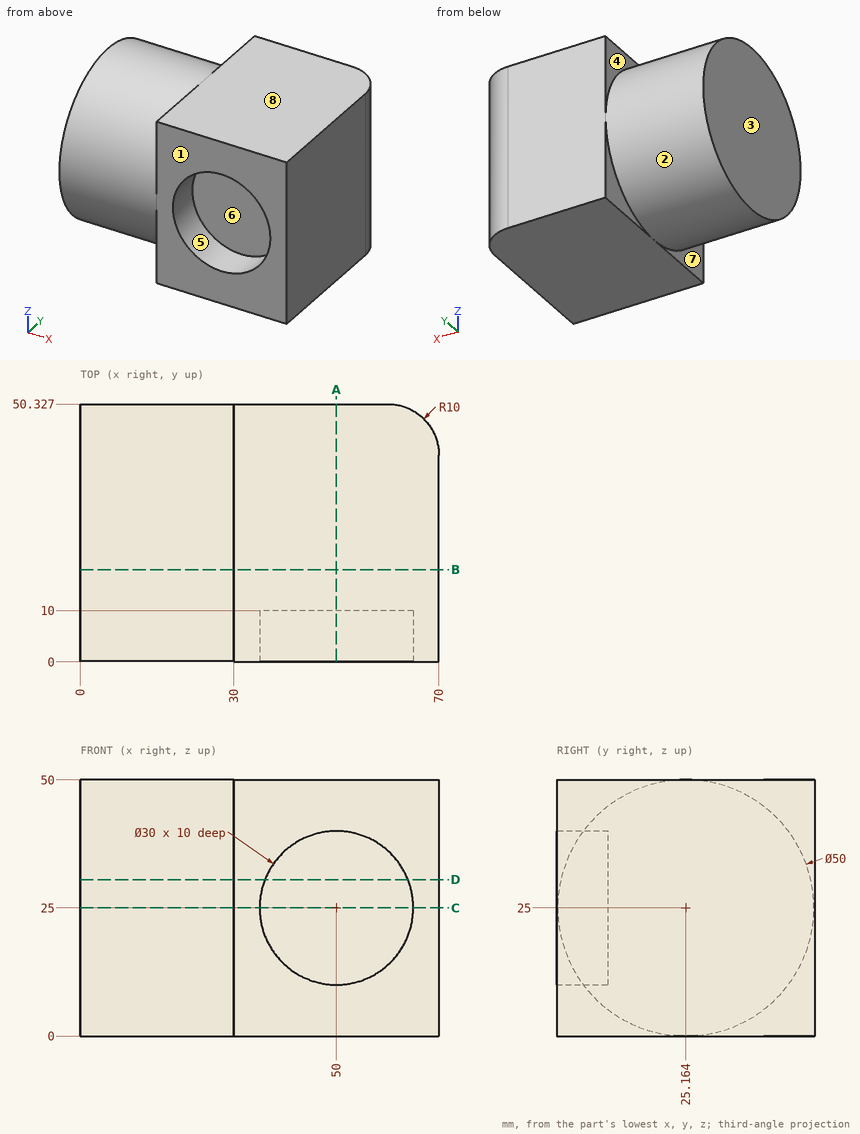
Check sheet for the drawn part. Datum: minimum x, y, z corner. Units: mm. A direction names the side the tool comes from. Coordinates: 2 decimals unless noted, no trailing zeros. Loops run counter-clockwise (first coordinate to the right, second up) from the corner with the lowest first, then second, coordinate; pieces in that order, holes last. Notation, with made-up numbers: (55.5, 61) -> (60.5, 61) arc R21 ccw to (60.5, 92) -> close; hole circle Ø10 at (49, 80). An arc over 180 degrees is marked (long way). Answer in a Markdown table with one row per item.
1. Sectioned sample at A-A, the plane x = 50. Record the boundary of the cut face in (y, z), then the cut area to 3 significant figures.
Check values:
| item | result |
|---|---|
| outline | (0, 0) -> (50.33, 0) -> (50.33, 50) -> (0, 50) -> (0, 40) -> (10, 40) -> (10, 10) -> (0, 10) -> close |
| area | 2,220 mm2 |
2. Release check for a two-part mould opening along Z. For the marked faces 6, 7 and 8 record: released by +Z, released by -Z, zero draft, split by the parting line, or undercut.
Check values:
| item | result |
|---|---|
| face 6 | undercut |
| face 7 | zero draft |
| face 8 | released by +Z |
3. Sectioned sample at D-D, the plane z = 30.5. Record the boundary of the cut face in (x, y) (1 decimal).
Check values:
| item | result |
|---|---|
| outline | (0, 0.8) -> (30, 0.8) -> (30, 0) -> (36, 0) -> (36, 10) -> (64, 10) -> (64, 0) -> (70, 0) -> (70, 40.3) arc R10 ccw to (60, 50.3) -> (30, 50.3) -> (30, 49.6) -> (0, 49.6) -> close |
4. Sectioned sample at C-C, the plane z = 25. Record the boundary of the cut face in (x, y).
Check values:
| item | result |
|---|---|
| outline | (0, 0.16) -> (30, 0.16) -> (30, 0) -> (35, 0) -> (35, 10) -> (65, 10) -> (65, 0) -> (70, 0) -> (70, 40.33) arc R10 ccw to (60, 50.33) -> (30, 50.33) -> (30, 50.16) -> (0, 50.16) -> close |
5. Access from +Z, -Z, +X, -X, +Y, -Y to the whole of each face (thin tool, end or side, straight path). Record for the marked faces 1, 2, 3, 4 and 5.
Check values:
| item | result |
|---|---|
| face 1 | +Z, -Z, +X, -X, -Y |
| face 2 | -X |
| face 3 | +Z, -Z, -X, +Y, -Y |
| face 4 | -X, +Y |
| face 5 | -Y |
6. Go/stop test with flat-tipped pins: pin 1 (10 mm diameter, centred on x = 22, y = 8, fed in from -Z); pin 2 (4 mm diameter, centred on x = 17, z = 38.5, fed in from +Y). Record where each tip stops, or that it passes through.
Check values:
| item | result |
|---|---|
| pin 1 | stops at z = 3.16 |
| pin 2 | stops at y = 47.36 |
7. Sectioned sample at B-B, the plane y = 18. Record the boundary of the cut face in (x, z), then the cut area to 3 significant figures.
Check values:
| item | result |
|---|---|
| outline | (0, 1.05) -> (30, 1.05) -> (30, 0) -> (70, 0) -> (70, 50) -> (30, 50) -> (30, 48.95) -> (0, 48.95) -> close |
| area | 3,440 mm2 |
8. Material ranges on line 1 along X through (y, z) = (2.75, 25); line 2 along Y through (x, z) = (62.5, 25.5); line 3 along X through (y, z) = (40, 47), recorded low to high. Write a range as [from, to].
Check values:
| item | result |
|---|---|
| line 1 | x = [0, 35], [65, 70] |
| line 2 | y = [10, 50.01] |
| line 3 | x = [30, 70] |
